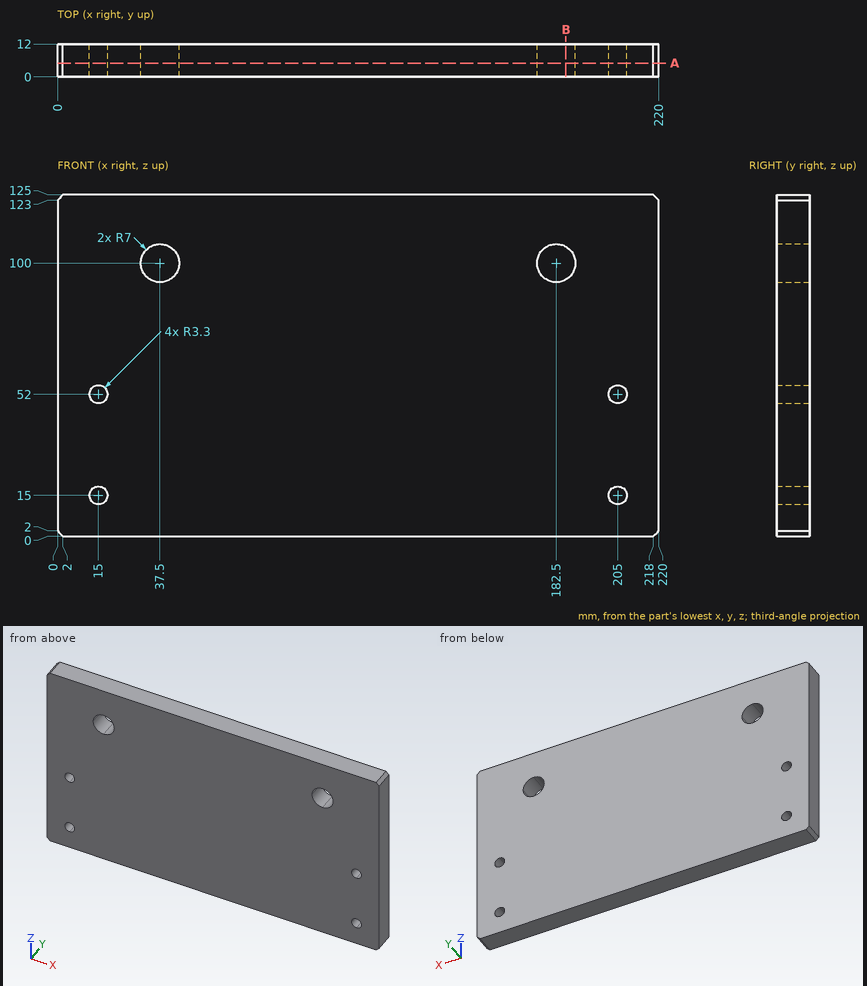
Answer from the drawing. Dimensions are ordinates in mm from the lowest x, y and z of the part. Coordinates: 2 decimals unless noted, no trailing zeros. Order: outer loops, then holes, each group sorted by start corner. A loop starts at its lowest first (then second) coordinate and runs counter-clockwise, first axis right, second up. Notation, with made-up numbers: (47, -31) - (57, -31) arc R31 cw to (57, 6) - close; hole circle Ø8 at (-12.5, 79.25). An arc over 180 degrees is marked (long way). Answer as a JSON object with one key per item and string values. Group by question number.
Item 1: Section A-A (y = 5) is taken. State how many separate pieces and enclosed holes the cut face has, plus the area to 3 significant figures.
Item 2: Section B-B (x = 186) is taken. Give the vertices of the cut face in (y, z), plus the area to 3 significant figures.
Item 3: Consider probe 1 along X at (y, z) = (4.5, 99.5); probe 2 along Z at (x, y) = (13, 9); probe 3 along X at (y, z) = (5.25, 17). Determine where each line is inside the solid, lowest interval first. Write a range as from..to.
Results are:
{
 "1": {"separate pieces": "1", "enclosed holes": "6", "area": "27,000 mm^2"},
 "2": {"outline": "(0, 0) - (12, 0) - (12, 93.94) - (0, 93.94) - close; (0, 106.06) - (12, 106.06) - (12, 125) - (0, 125) - close", "area": "1,350 mm^2"},
 "3": {"probe 1": "x = 0..30.52, 44.48..175.52, 189.48..220", "probe 2": "z = 0..12.38, 17.62..49.38, 54.62..125", "probe 3": "x = 0..12.38, 17.62..202.38, 207.62..220"}
}
